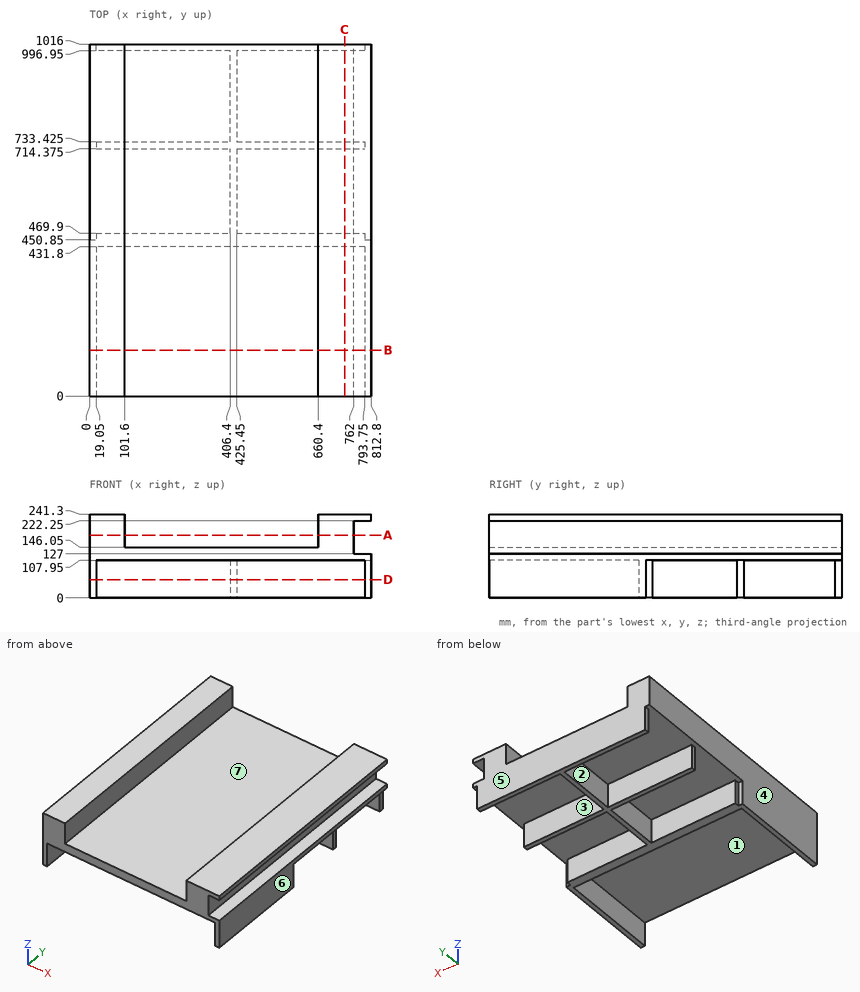
Part print with two shaded views. Sizes in mm from the minimum x, y, z corner. A direction names the side the tool comes from. Coordinates: 2 decimals unless noted, no trailing zeros. Order: outer loops, then holes, each group sorted by start corner. A loop starts at its lowest first (then second) coordinate and runs counter-clockwise, first axis right, second up.
(1) Saw through at A-A, the plane z = 181. Write the cut outline in (x, y).
Solution:
outline: (0, 0) - (101.6, 0) - (101.6, 1016) - (0, 1016) - close; (660.4, 0) - (762, 0) - (762, 1016) - (660.4, 1016) - close
(2) Pin check, flat tips, straight feed: pin 1 Ø2 at (x, z) = (538, 74.5) entering from -Y; pin 2 Ø2 at (y, z) = (196, 133.5) entering from +X; pin 3 Ø6 at (x, y) = (564.5, 157.5) entering from +Z. Stop position of each tip, or through.
Solution:
pin 1: stops at y = 431.8
pin 2: stops at x = 762
pin 3: stops at z = 146.05
(3) Saw through at C-C, the plane x = 736. Write the cut outline in (y, z) (3 decimals).
Solution:
outline: (0, 107.95) - (431.8, 107.95) - (431.8, 0) - (469.9, 0) - (469.9, 107.95) - (714.375, 107.95) - (714.375, 0) - (733.425, 0) - (733.425, 107.95) - (996.95, 107.95) - (996.95, 0) - (1016, 0) - (1016, 241.3) - (0, 241.3) - close
(4) Drill centre lines: L1, parallel to Y at x = 376.5, z = 98 (3 decimals); L2, parallel to X at y = 732, z = 198; L3, parallel to X at y = 423, z = 105. Where is each one in solid material? Low to high.
Solution:
L1: y = 431.8 to 469.9, 714.375 to 733.425, 996.95 to 1016
L2: x = 0 to 101.6, 660.4 to 762
L3: x = 0 to 19.05, 793.75 to 812.8
(5) Saw through at D-D, the plane z = 53. Write the cut outline in (x, y) (3 decimals), and give its area (3 significant figures).
Solution:
outline: (0, 0) - (19.05, 0) - (19.05, 431.8) - (793.75, 431.8) - (793.75, 0) - (812.8, 0) - (812.8, 450.85) - (793.75, 450.85) - (793.75, 469.9) - (425.45, 469.9) - (425.45, 714.375) - (793.75, 714.375) - (793.75, 733.425) - (425.45, 733.425) - (425.45, 996.95) - (793.75, 996.95) - (793.75, 1016) - (19.05, 1016) - (19.05, 996.95) - (406.4, 996.95) - (406.4, 733.425) - (19.05, 733.425) - (19.05, 714.375) - (406.4, 714.375) - (406.4, 469.9) - (19.05, 469.9) - (19.05, 450.85) - (0, 450.85) - close
area: 85,900 mm2
(6) Which spindle directions (+Z, -Z, +X, -X, +Y, -Y) get a long thin tool onto all of the face, cutting with end or side? Do the marked faces 1, 2 and 3. Say none if no direction does.
Solution:
face 1: -Z, -Y
face 2: -Z, -X
face 3: -Z, +X
(7) Mould opens along X. For the marked faces 4, 5, 6 and 7 say: released by +X, released by -X, zero draft, split by the parting line, or undercut.
Solution:
face 4: released by -X
face 5: zero draft
face 6: released by +X
face 7: undercut
(8) Saw through at B-B, the plane y = 133. Write the cut outline in (x, z), and give its area (3 significant figures).
Solution:
outline: (0, 0) - (19.05, 0) - (19.05, 107.95) - (793.75, 107.95) - (793.75, 0) - (812.8, 0) - (812.8, 127) - (762, 127) - (762, 222.25) - (812.8, 222.25) - (812.8, 241.3) - (660.4, 241.3) - (660.4, 146.05) - (101.6, 146.05) - (101.6, 241.3) - (0, 241.3) - close
area: 54,400 mm2
